Job drawing, mm, ordinate dimensions from the low corner. One solid piece. A direction names the side the tool comes from. Give positions to 0.01 mm unless a question says otherwise; leave off trailing zeros. Loops run counter-clockwise (first coordinate to the right, second up) from the corner with the lowest first, then second, coordinate; pieces in that order, holes last. Notation, with made-up numbers: (77, -21) -> (93, -21) arc R32 cw to (93, 14) -> close; hole circle Ø7 at (87.5, 2.5). An arc over 180 degrees is marked (long way). Use one line per item in the form item = value.
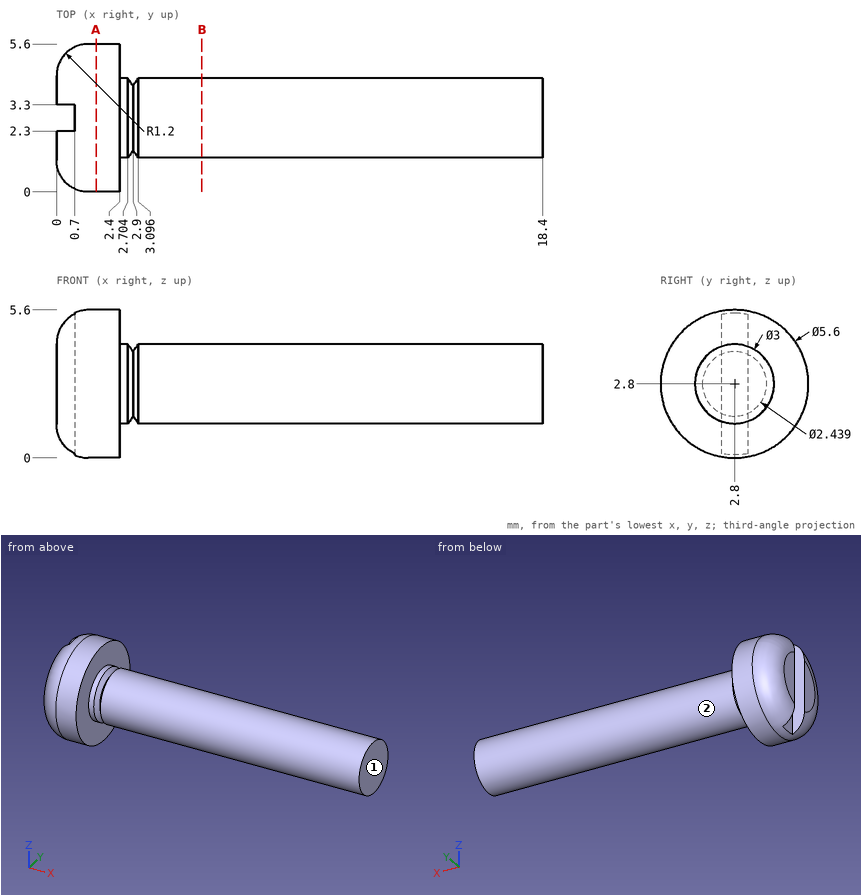
1. Tool access for the marked faces 1 and 2: list every direction of +Z, -Z, +X, -X, +Y, -Y with a clear straight run to the whole face (end or side of a thin tool).
Result sheet:
face_1 = +Z, -Z, +X, +Y, -Y
face_2 = +X
2. Cut at B-B, the plane x = 5.5. Write the cut outline in (y, z).
Result sheet:
outline = circle Ø3 at (2.8, 2.8)
3. Drop flat-ended pins along their axis: P1, Ø2, axis at x = 2, y = 2, coming from the -Z side; P2, Ø3, axis at x = 12, y = 3, coming from the -Z side. Give the stop position or say it passes through.
Result sheet:
P1 = 0
P2 = 1.3
4. Drill centre lines: line 1 (X direction, y = 1.95, z = 1.35); line 2 (Z direction, x = 17.5, y = 2.85); line 3 (X direction, y = 3.15, z = 3.3). Where is each one in solid material? Low to high.
Result sheet:
line_1 = 0 to 2.4
line_2 = 1.3 to 4.3
line_3 = 0.7 to 18.4
5. Cut at A-A, the plane x = 1.5. Write the cut outline in (y, z), then the cut area to 3 significant figures.
Result sheet:
outline = circle Ø5.6 at (2.8, 2.8)
area = 24.6 mm^2
